Input: part model. Units: mm. Frame: model coordinates. A direction names the side the tool comes from. Round coordinates to 2 decimals unless told otherwise and drop trailing zeros. Loops run counter-clockwise (first coordinate to the right, second up) from the corner with the lowest first, then second, coordinate; pieces in that order, holes last. Notation, with made-up numbers: (-19, 6.5) -> (13, 6.5) arc R4 ccw to (13, 12.5) -> close; hole circle Ø10 at (66.5, 16.5). An arc over 180 degrees is marked (long way). Answer as a JSON object with one key per item and string values. Group by question number.
Item 1: Section query B-B on x = 7. Return loops of the section in (y, z), and give its area (3 significant figures).
Item 2: Set-up query: faces 4 (the flat face through (13.8, -1, 12)), 5 (the cylindrical face through (-12.476, -0.74, -14.744)), 6 (the flat face through (21, 1, -7.6)). Return all of +Z, -Z, +X, -X, +Y, -Y with unobstructed straight access to the full face (end or side cutting, diameter ignored); none if empty.
Item 3: Section query C-C on z = 0. Return loops of the section in (x, y).
Item 4: Section query A-A on z = -8.5. Return loops of the section in (x, y), and give its area (3 significant figures).
Item 5: Pin query (flat end, axial travel): pin 1 (0.7 mm diameter, centred on y = 5, z = -11.5, fed in from -X); pin 2 (8 mm diameter, centred on x = -4.5, z = -3.5, fed in from +Y); pin 3 (2 mm diameter, centred on x = 20.8, z = -12.1, fed in from +Y); pin 4 (1.2 mm diameter, centred on y = -1, z = -13.5, fed in from -X). Return the tip coordinate at first contact, or that it passes through.
Item 6: Draft query along X for faces 1 (the flat face through (-16, -1, 13.4)), 2 (the cylindrical face through (-25.4, 3.35, -0.05)), 3 (the flat face through (-21, 1.75, 8)). Return one class per face: released by +X, released by -X, zero draft, split by the parting line, or undercut.
Item 7: Material intervals for line 1 (Z direction, x = -20.8, y = 3); line 2 (X direction, y = 4.75, z = 12.1); line 3 (Z direction, x = 15, y = 2.25), sorted ascending. Write a range as [from, to].
from build123d import *

# Parameters (mm, degrees)
SKETCH1_W           = 43.8
SKETCH1_H           = 18.2
SKETCH1_R           = 1.1
BOSS_EXTRUDE1_DEPTH = 7.6
SKETCH3_R           = 1.1
BOSS_EXTRUDE2_DEPTH = 1.5
CUT_EXTRUDE1_REACH  = 54.6
SKETCH5_W           = 1.5
SKETCH5_H           = 1.5
BOSS_EXTRUDE3_DEPTH = 1.75
CUT_EXTRUDE2_REACH  = 54.6
BOSS_EXTRUDE4_DEPTH = 1.5
FILLET1_R           = 1.25
FILLET2_R           = 0.5


with BuildPart() as part:
    # Sketch1 → Boss-Extrude1 (new body)
    with BuildSketch(Plane(origin=(0, 0, 0), x_dir=(1, 0, 0), z_dir=(0, 1, 0))):
        with BuildLine():
            ThreePointArc((-23.8, -12.1), (-20.8, -15.1), (-17.8, -12.1))
            Line((-17.8, -12.1), (-17.8, -11))
            Line((-17.8, -11), (17.8, -11))
            Line((17.8, -11), (17.8, -12.1))
            ThreePointArc((17.8, -12.1), (20.8, -15.1), (23.8, -12.1))
            Line((23.8, -12.1), (23.8, 12.1))
            ThreePointArc((23.8, 12.1), (20.8, 15.1), (17.8, 12.1))
            Line((17.8, 12.1), (17.8, 11))
            Line((17.8, 11), (-17.8, 11))
            Line((-17.8, 11), (-17.8, 12.1))
            ThreePointArc((-17.8, 12.1), (-20.8, 15.1), (-23.8, 12.1))
            Line((-23.8, 12.1), (-23.8, 4))
            Line((-23.8, 4), (-28.8, 4))
            Line((-28.8, 4), (-28.8, -4))
            Line((-28.8, -4), (-23.8, -4))
            Line((-23.8, -4), (-23.8, -12.1))
        make_face()
        Rectangle(SKETCH1_W, SKETCH1_H, mode=Mode.SUBTRACT)
        with Locations((-20.8, 12.1)):
            Circle(SKETCH1_R, mode=Mode.SUBTRACT)
        with Locations((20.8, 12.1)):
            Circle(SKETCH1_R, mode=Mode.SUBTRACT)
        with Locations((-20.8, -12.1)):
            Circle(SKETCH1_R, mode=Mode.SUBTRACT)
        with Locations((20.8, -12.1)):
            Circle(SKETCH1_R, mode=Mode.SUBTRACT)
    extrude(amount=BOSS_EXTRUDE1_DEPTH)

    # Sketch3 → Boss-Extrude2 (add)
    with BuildSketch(Plane.XZ):
        with BuildLine():
            Line((-23.8, -4), (-23.8, -12.1))
            ThreePointArc((-23.8, -12.1), (-20.8, -15.1), (-17.8, -12.1))
            Line((-17.8, -12.1), (-17.8, -11))
            Line((-17.8, -11), (17.8, -11))
            Line((17.8, -11), (17.8, -12.1))
            ThreePointArc((17.8, -12.1), (20.8, -15.1), (23.8, -12.1))
            Line((23.8, -12.1), (23.8, 12.1))
            ThreePointArc((23.8, 12.1), (20.8, 15.1), (17.8, 12.1))
            Line((17.8, 12.1), (17.8, 11))
            Line((17.8, 11), (-17.8, 11))
            Line((-17.8, 11), (-17.8, 12.1))
            ThreePointArc((-17.8, 12.1), (-20.8, 15.1), (-23.8, 12.1))
            Line((-23.8, 12.1), (-23.8, 4))
            Line((-23.8, 4), (-28.8, 4))
            Line((-28.8, 4), (-28.8, -4))
            Line((-28.8, -4), (-23.8, -4))
        make_face()
        with Locations((-20.8, -12.1)):
            Circle(SKETCH3_R, mode=Mode.SUBTRACT)
        with Locations((20.8, -12.1)):
            Circle(SKETCH3_R, mode=Mode.SUBTRACT)
        with Locations((20.8, 12.1)):
            Circle(SKETCH3_R, mode=Mode.SUBTRACT)
        with Locations((-20.8, 12.1)):
            Circle(SKETCH3_R, mode=Mode.SUBTRACT)
    extrude(amount=BOSS_EXTRUDE2_DEPTH)

    # Sketch4 → Cut-Extrude1 (cut, up to next)
    with BuildSketch(Plane.ZY.offset(28.8), mode=Mode.PRIVATE) as cut_extrude1_sk1:
        with BuildLine():
            Line((-2.25, 7.6), (-2.25, 5.6))
            ThreePointArc((-2.25, 5.6), (0, 3.35), (2.25, 5.6))
            Line((2.25, 5.6), (2.25, 7.6))
            Line((2.25, 7.6), (-2.25, 7.6))
        make_face()
    cut_extrude1_tool1 = extrude(cut_extrude1_sk1.sketch, amount=-CUT_EXTRUDE1_REACH, mode=Mode.PRIVATE) & part.part
    add(cut_extrude1_tool1.solids().sort_by_distance((-28.8, 5.682954, 0))[0], mode=Mode.SUBTRACT)

    # Sketch5 → Boss-Extrude3 (add)
    with BuildSketch(Plane(origin=(0, 0, 0), x_dir=(1, 0, 0), z_dir=(0, 1, 0))):
        with Locations((-21.15, 8.35)):
            Rectangle(SKETCH5_W, SKETCH5_H)
        with Locations((21.15, 8.35)):
            Rectangle(SKETCH5_W, SKETCH5_H)
        with Locations((-21.15, -8.35)):
            Rectangle(SKETCH5_W, SKETCH5_H)
        with Locations((21.15, -8.35)):
            Rectangle(SKETCH5_W, SKETCH5_H)
    extrude(amount=BOSS_EXTRUDE3_DEPTH)

    # Sketch6 → Cut-Extrude2 (cut, up to next)
    with BuildSketch(Plane(origin=(23.8, 0, 0), x_dir=(0, 0, -1), z_dir=(1, 0, 0)), mode=Mode.PRIVATE) as cut_extrude2_sk1:
        Polygon((3.8, 7.6), (-3.8, 7.6), (-3.8, 5.5), (-3.5, 5.2), (-3.5, 3.8), (3.5, 3.8), (3.5, 5.2), (3.8, 5.5), align=None)
    cut_extrude2_tool1 = extrude(cut_extrude2_sk1.sketch, amount=-CUT_EXTRUDE2_REACH, mode=Mode.PRIVATE) & part.part
    add(cut_extrude2_tool1.solids().sort_by_distance((23.8, 5.737352, 0))[0], mode=Mode.SUBTRACT)

    # Sketch8 → Boss-Extrude4 (add)
    with BuildSketch(Plane.XZ.offset(1.5)):
        with BuildLine():
            Line((-12.1, 15.1), (-20.8, 15.1))
            ThreePointArc((-20.8, 15.1), (-18.678679656, 14.221320344), (-17.8, 12.1))
            Line((-17.8, 12.1), (-17.8, 13.4))
            Line((-17.8, 13.4), (-13.8, 13.4))
            Line((-13.8, 13.4), (-13.8, 11))
            Line((-13.8, 11), (-12.1, 11))
            Line((-12.1, 11), (-12.1, 15.1))
        make_face()
        with BuildLine():
            Line((12.1, 15.1), (12.1, 11))
            Line((12.1, 11), (13.8, 11))
            Line((13.8, 11), (13.8, 13.4))
            Line((13.8, 13.4), (17.8, 13.4))
            Line((17.8, 13.4), (17.8, 12.1))
            ThreePointArc((17.8, 12.1), (18.678679656, 14.221320344), (20.8, 15.1))
            Line((20.8, 15.1), (12.1, 15.1))
        make_face()
        with BuildLine():
            Line((13.8, -11), (12.1, -11))
            Line((12.1, -11), (12.1, -15.1))
            Line((12.1, -15.1), (20.8, -15.1))
            ThreePointArc((20.8, -15.1), (18.678679656, -14.221320344), (17.8, -12.1))
            Line((17.8, -12.1), (17.8, -13.4))
            Line((17.8, -13.4), (13.8, -13.4))
            Line((13.8, -13.4), (13.8, -11))
        make_face()
        with BuildLine():
            Line((-20.8, -15.1), (-12.1, -15.1))
            Line((-12.1, -15.1), (-12.1, -11))
            Line((-12.1, -11), (-13.8, -11))
            Line((-13.8, -11), (-13.8, -13.4))
            Line((-13.8, -13.4), (-17.8, -13.4))
            Line((-17.8, -13.4), (-17.8, -12.1))
            ThreePointArc((-17.8, -12.1), (-18.678679656, -14.221320344), (-20.8, -15.1))
        make_face()
    extrude(amount=-BOSS_EXTRUDE4_DEPTH)

    # Fillet1
    fillet1_edges = [part.edges().sort_by_distance(p)[0] for p in [
        (-12.1, -0.75, 15.1),
        (-12.1, -0.75, 11),
        (12.1, -0.75, 11),
        (12.1, -0.75, 15.1),
        (12.1, -0.75, -15.1),
        (12.1, -0.75, -11),
        (-12.1, -0.75, -11),
        (-12.1, -0.75, -15.1),
        (-23.8, 3.05, 4),
        (-28.8, 3.05, 4),
        (-28.8, 3.05, -4),
        (-23.8, 3.05, -4),
    ]]
    fillet(fillet1_edges, radius=FILLET1_R)

    # Fillet2
    fillet2_edges = [part.edges().sort_by_distance(p)[0] for p in [
        (22.85, 5.2, -3.5),
        (22.85, 3.8, -3.5),
        (22.85, 3.8, 3.5),
        (22.85, 5.2, 3.5),
        (22.85, 5.5, 3.8),
        (22.85, 5.5, -3.8),
    ]]
    fillet(fillet2_edges, radius=FILLET2_R)


solid = part.part
Solved:
{
 "1": {"outline": "(-1.5, -11) -> (7.6, -11) -> (7.6, -9.1) -> (0, -9.1) -> (0, 9.1) -> (7.6, 9.1) -> (7.6, 11) -> (-1.5, 11) -> close", "area": "61.9 mm²"},
 "2": {"face 4": "+Y, -Y", "face 5": "-Z, +Y, -Y", "face 6": "+Y"},
 "3": {"outline": "(-28.8, -1.5) -> (23.8, -1.5) -> (23.8, 3.8) -> (21.9, 3.8) -> (21.9, 0) -> (-21.9, 0) -> (-21.9, 3.35) -> (-28.8, 3.35) -> close"},
 "4": {"outline": "(-23.8, -1.5) -> (23.8, -1.5) -> (23.8, 7.6) -> (21.9, 7.6) -> (21.9, 1.75) -> (20.4, 1.75) -> (20.4, 0) -> (-20.4, 0) -> (-20.4, 1.75) -> (-21.9, 1.75) -> (-21.9, 7.6) -> (-23.8, 7.6) -> close", "area": "106 mm²"},
 "5": {"pin 1": "x = -23.8", "pin 2": "y = 0", "pin 3": "through", "pin 4": "x = -23.69"},
 "6": {"face 1": "undercut", "face 2": "zero draft", "face 3": "undercut"},
 "7": {"line 1": "[-15.1, -13.2], [-11, -9.1], [9.1, 11], [13.2, 15.1]", "line 2": "[-23.8, -21.9], [-19.7, -17.8], [17.8, 19.7], [21.9, 23.8]", "line 3": "[-11, -9.1], [9.1, 11]"}
}
